from build123d import *

# Parameters (mm, degrees)
SKETCH2_W                   = 150
SKETCH2_H                   = 25
BASE_FLANGE1_DEPTH          = 0.9
F_19_0_166_DIAMETER_SLOT1_D = 4.2164
F_19_0_166_DIAMETER_SLOT2_D = 4.2164
F_1_0MM_DOWEL_SLOT1_D       = 3.5


# Sheet-metal steps are written as plain solids
with BuildPart() as part:
    # Sketch2 → Base-Flange1 (new body)
    with BuildSketch(Plane.XY):
        Rectangle(SKETCH2_W, SKETCH2_H)
    extrude(amount=-BASE_FLANGE1_DEPTH)

    # #19 (0.166) Diameter Slot1 (through all)
    with Locations(Plane(origin=(0, 0, -0.9), x_dir=(-1, 0, 0), z_dir=(0, 0, -1))):
        with Locations((-64.628032866, 0)):
            Hole(F_19_0_166_DIAMETER_SLOT1_D / 2)

    # #19 (0.166) Diameter Slot2 (through all)
    with Locations(Plane.XY):
        with Locations((-66.567919304, 8.5), (-66.567919304, -8.5)):
            Hole(F_19_0_166_DIAMETER_SLOT2_D / 2)

    # Ø1.0mm Dowel Slot1 (through all)
    with Locations(Plane.XY):
        with Locations((47.178032866, 0)):
            Hole(F_1_0MM_DOWEL_SLOT1_D / 2)


solid = part.part
The listing builds one solid part. Answer for the finished solid, in the listing's coordinates (mm). Round coordinates to 2 decimals unless told otherwise and drop trailing zeros. Order: outer loops, then holes, each group sorted by start corner. A loop starts at its lowest first (then second) coordinate and runs counter-clockwise, first axis right, second up. Notation, with made-up numbers: M 37.5,87.25 L 46.5,87.25 A32 ccw 46.5,116.25 Z; hole C 88.25,77 d9. An arc over 180 degrees is marked long. Answer in a Markdown table with one row per item. Add a question column.
1) Determine the mould class of faces 1 (the face through (48.926, 0.077, -0.456)), 2 (the face through (-1, 0, -0.9)) for opening direction Y: pulls with the +Y half, pulls with the -Y half, needs draft (parallel to the pull), parting line crosses it, or undercut.
2) Consider line 1 along X through (y, z) = (9.25, -0.35); line 2 along X through (y, z) = (7, -0.8); line 3 along Y through (x, z) = (63, -0.5). Determine where each line is inside the solid, lowest interval first. Write a range as from..to.
3) The part is cut by section A-A on y = 0. Determine the outline of the cut face in (x, z).
4) The part is cut by section B-B on y = -8.5. Determine the outline of the cut face in (x, z), plus the area to 3 significant figures.
Findings below:
| question | item | result |
|---|---|---|
| 1 | face 1 | undercut |
| 1 | face 2 | needs draft |
| 2 | line 1 | x = -75..-68.54, -64.6..75 |
| 2 | line 2 | x = -75..-68.05, -65.09..75 |
| 2 | line 3 | y = -12.5..-1.34, 1.34..12.5 |
| 3 | outline | M -75,-0.9 L 45.43,-0.9 L 45.43,0 L -75,0 Z; M 48.93,-0.9 L 62.52,-0.9 L 62.52,0 L 48.93,0 Z; M 66.74,-0.9 L 75,-0.9 L 75,0 L 66.74,0 Z |
| 4 | outline | M -75,-0.9 L -68.68,-0.9 L -68.68,0 L -75,0 Z; M -64.46,-0.9 L 75,-0.9 L 75,0 L -64.46,0 Z |
| 4 | area | 131 mm² |
